```python
from build123d import *

# Parameters (mm, degrees)
SKETCH1_R           = 3.95
SKETCH1_R_2         = 1.975
SKETCH1_R_3         = 1.475
SKETCH1_W           = 10
SKETCH1_H           = 5
BOSS_EXTRUDE1_DEPTH = 5


with BuildPart() as part:
    # Sketch1 → Boss-Extrude1 (new body)
    with BuildSketch(Plane.XY):
        with BuildLine():
            Line((-19, 0), (-19, 130))
            ThreePointArc((-19, 130), (0, 149), (19, 130))
            Line((19, 130), (19, 0))
            ThreePointArc((19, 0), (0, -19), (-19, 0))
        make_face()
        Circle(SKETCH1_R, mode=Mode.SUBTRACT)
        with Locations((0, 12)):
            Circle(SKETCH1_R_2, mode=Mode.SUBTRACT)
        with Locations((12, 0)):
            Circle(SKETCH1_R_2, mode=Mode.SUBTRACT)
        with Locations((0, -12)):
            Circle(SKETCH1_R_2, mode=Mode.SUBTRACT)
        with Locations((-12, 0)):
            Circle(SKETCH1_R_2, mode=Mode.SUBTRACT)
        with Locations((13.5, 25)):
            Circle(SKETCH1_R_3, mode=Mode.SUBTRACT)
        with Locations((4.5, 25)):
            Circle(SKETCH1_R_3, mode=Mode.SUBTRACT)
        with Locations((13.5, 31.5)):
            Circle(SKETCH1_R_3, mode=Mode.SUBTRACT)
        with Locations((4.5, 31.5)):
            Circle(SKETCH1_R_3, mode=Mode.SUBTRACT)
        with Locations((13.5, 18.5)):
            Circle(SKETCH1_R_3, mode=Mode.SUBTRACT)
        with Locations((4.5, 18.5)):
            Circle(SKETCH1_R_3, mode=Mode.SUBTRACT)
        with Locations((0, 122.5)):
            Circle(SKETCH1_R_3, mode=Mode.SUBTRACT)
        with BuildLine():
            Line((7.5, 103.5), (7.5, 90.5))
            ThreePointArc((7.5, 90.5), (4.5, 87.5), (1.5, 90.5))
            Line((1.5, 90.5), (1.5, 103.5))
            ThreePointArc((1.5, 103.5), (4.5, 106.5), (7.5, 103.5))
        make_face(mode=Mode.SUBTRACT)
        with BuildLine():
            Line((-7.5, 103.5), (-7.5, 90.5))
            ThreePointArc((-7.5, 90.5), (-4.5, 87.5), (-1.5, 90.5))
            Line((-1.5, 90.5), (-1.5, 103.5))
            ThreePointArc((-1.5, 103.5), (-4.5, 106.5), (-7.5, 103.5))
        make_face(mode=Mode.SUBTRACT)
        with BuildLine():
            Line((16.5, 103.5), (16.5, 90.5))
            ThreePointArc((16.5, 90.5), (13.5, 87.5), (10.5, 90.5))
            Line((10.5, 90.5), (10.5, 103.5))
            ThreePointArc((10.5, 103.5), (13.5, 106.5), (16.5, 103.5))
        make_face(mode=Mode.SUBTRACT)
        with BuildLine():
            Line((-16.5, 103.5), (-16.5, 90.5))
            ThreePointArc((-16.5, 90.5), (-13.5, 87.5), (-10.5, 90.5))
            Line((-10.5, 90.5), (-10.5, 103.5))
            ThreePointArc((-10.5, 103.5), (-13.5, 106.5), (-16.5, 103.5))
        make_face(mode=Mode.SUBTRACT)
        with BuildLine():
            Line((7.5, 79.5), (7.5, 66.5))
            ThreePointArc((7.5, 66.5), (4.5, 63.5), (1.5, 66.5))
            Line((1.5, 66.5), (1.5, 79.5))
            ThreePointArc((1.5, 79.5), (4.5, 82.5), (7.5, 79.5))
        make_face(mode=Mode.SUBTRACT)
        with BuildLine():
            Line((-7.5, 79.5), (-7.5, 66.5))
            ThreePointArc((-7.5, 66.5), (-4.5, 63.5), (-1.5, 66.5))
            Line((-1.5, 66.5), (-1.5, 79.5))
            ThreePointArc((-1.5, 79.5), (-4.5, 82.5), (-7.5, 79.5))
        make_face(mode=Mode.SUBTRACT)
        with BuildLine():
            Line((16.5, 79.5), (16.5, 66.5))
            ThreePointArc((16.5, 66.5), (13.5, 63.5), (10.5, 66.5))
            Line((10.5, 66.5), (10.5, 79.5))
            ThreePointArc((10.5, 79.5), (13.5, 82.5), (16.5, 79.5))
        make_face(mode=Mode.SUBTRACT)
        with BuildLine():
            Line((-16.5, 79.5), (-16.5, 66.5))
            ThreePointArc((-16.5, 66.5), (-13.5, 63.5), (-10.5, 66.5))
            Line((-10.5, 66.5), (-10.5, 79.5))
            ThreePointArc((-10.5, 79.5), (-13.5, 82.5), (-16.5, 79.5))
        make_face(mode=Mode.SUBTRACT)
        with BuildLine():
            Line((7.5, 55.5), (7.5, 42.5))
            ThreePointArc((7.5, 42.5), (4.5, 39.5), (1.5, 42.5))
            Line((1.5, 42.5), (1.5, 55.5))
            ThreePointArc((1.5, 55.5), (4.5, 58.5), (7.5, 55.5))
        make_face(mode=Mode.SUBTRACT)
        with BuildLine():
            Line((-7.5, 55.5), (-7.5, 42.5))
            ThreePointArc((-7.5, 42.5), (-4.5, 39.5), (-1.5, 42.5))
            Line((-1.5, 42.5), (-1.5, 55.5))
            ThreePointArc((-1.5, 55.5), (-4.5, 58.5), (-7.5, 55.5))
        make_face(mode=Mode.SUBTRACT)
        with BuildLine():
            Line((16.5, 55.5), (16.5, 42.5))
            ThreePointArc((16.5, 42.5), (13.5, 39.5), (10.5, 42.5))
            Line((10.5, 42.5), (10.5, 55.5))
            ThreePointArc((10.5, 55.5), (13.5, 58.5), (16.5, 55.5))
        make_face(mode=Mode.SUBTRACT)
        with BuildLine():
            Line((-16.5, 55.5), (-16.5, 42.5))
            ThreePointArc((-16.5, 42.5), (-13.5, 39.5), (-10.5, 42.5))
            Line((-10.5, 42.5), (-10.5, 55.5))
            ThreePointArc((-10.5, 55.5), (-13.5, 58.5), (-16.5, 55.5))
        make_face(mode=Mode.SUBTRACT)
        with BuildLine():
            Line((-7.5, 31.5), (-7.5, 18.5))
            ThreePointArc((-7.5, 18.5), (-4.5, 15.5), (-1.5, 18.5))
            Line((-1.5, 18.5), (-1.5, 31.5))
            ThreePointArc((-1.5, 31.5), (-4.5, 34.5), (-7.5, 31.5))
        make_face(mode=Mode.SUBTRACT)
        with BuildLine():
            Line((-16.5, 31.5), (-16.5, 18.5))
            ThreePointArc((-16.5, 18.5), (-13.5, 15.5), (-10.5, 18.5))
            Line((-10.5, 18.5), (-10.5, 31.5))
            ThreePointArc((-10.5, 31.5), (-13.5, 34.5), (-16.5, 31.5))
        make_face(mode=Mode.SUBTRACT)
        with Locations((10, 122.5)):
            Rectangle(SKETCH1_W, SKETCH1_H, mode=Mode.SUBTRACT)
        with Locations((-10, 122.5)):
            Rectangle(SKETCH1_W, SKETCH1_H, mode=Mode.SUBTRACT)
    extrude(amount=BOSS_EXTRUDE1_DEPTH)


solid = part.part
```
The model under review builds one solid part; all positions refer to its coordinate system, in mm. Round coordinates to 2 decimals unless told otherwise and drop trailing zeros. Loops run counter-clockwise (first coordinate to the right, second up) from the corner with the lowest first, then second, coordinate; pieces in that order, holes last. Notation, with made-up numbers: (-18, 82.25) -> (-8, 82.25) arc R18 ccw to (-8, 89.25) -> close; hole circle Ø7 at (-26, 27). An arc over 180 degrees is marked (long way). Answer as a JSON object with one key per item and string values. Group by question number.
1) We need section C-C on z = 4.2. Give the number of separate pieces and of enclosed holes in the cut face, then the cut area to 3 significant figures.
2) For pin 1 Ø2 at (x, z) = (11.5, 4) entering from -Y; pin 2 Ø1.5 at (x, z) = (9, 2) entering from -Y; pin 3 Ø2.5 at (x, y) = (4.5, 18.5) entering from -Z, all flat-tipped, find the tip position at first contact; note any pin that passes through.
3) We need section B-B on x = -12. Write out the cut boundary in (y, z) (3 decimals), then the cut area to 3 significant figures.
4) We need section A-A on x = 0. Write out the cut boundary in (y, z) (3 decimals), then the cut area to 3 significant figures.
5) For line 1 (Y direction, x = 0, z = 1.35) (3 decimals); line 2 (X direction, y = 101, z = 4.55); line 3 (X direction, y = 122.5, z = 2.7) (3 decimals), list the stretches that pass through material, from the lowest coordinate up. Write a range as [from, to].
6) We need section D-D on y = 134. Write out the cut boundary in (x, z).
7) Mouldability with a two-part tool opening along Y and no side actions: class faces 1 (the face through (0, 66, 5)), 2 (the face through (4.4, 106.5, 2.5)) as released by +Y, released by -Y, zero draft, split by the parting line, or undercut.
Result set:
{
 "1": {"separate pieces": "1", "enclosed holes": "28", "area": "4,340 mm²"},
 "2": {"pin 1": "y = -15.84", "pin 2": "y = -17.12", "pin 3": "through"},
 "3": {"outline": "(-14.731, 0) -> (-1.975, 0) -> (-1.975, 5) -> (-14.731, 5) -> close; (1.975, 0) -> (15.902, 0) -> (15.902, 5) -> (1.975, 5) -> close; (34.098, 0) -> (39.902, 0) -> (39.902, 5) -> (34.098, 5) -> close; (58.098, 0) -> (63.902, 0) -> (63.902, 5) -> (58.098, 5) -> close; (82.098, 0) -> (87.902, 0) -> (87.902, 5) -> (82.098, 5) -> close; (106.098, 0) -> (120, 0) -> (120, 5) -> (106.098, 5) -> close; (125, 0) -> (144.731, 0) -> (144.731, 5) -> (125, 5) -> close", "area": "389 mm²"},
 "4": {"outline": "(-19, 0) -> (-13.975, 0) -> (-13.975, 5) -> (-19, 5) -> close; (-10.025, 0) -> (-3.95, 0) -> (-3.95, 5) -> (-10.025, 5) -> close; (3.95, 0) -> (10.025, 0) -> (10.025, 5) -> (3.95, 5) -> close; (13.975, 0) -> (121.025, 0) -> (121.025, 5) -> (13.975, 5) -> close; (123.975, 0) -> (149, 0) -> (149, 5) -> (123.975, 5) -> close", "area": "746 mm²"},
 "5": {"line 1": "[-19, -13.975], [-10.025, -3.95], [3.95, 10.025], [13.975, 121.025], [123.975, 149]", "line 2": "[-19, -16.5], [-10.5, -7.5], [-1.5, 1.5], [7.5, 10.5], [16.5, 19]", "line 3": "[-19, -15], [-5, -1.475], [1.475, 5], [15, 19]"},
 "6": {"outline": "(-18.57, 0) -> (18.57, 0) -> (18.57, 5) -> (-18.57, 5) -> close"},
 "7": {"face 1": "zero draft", "face 2": "undercut"}
}
